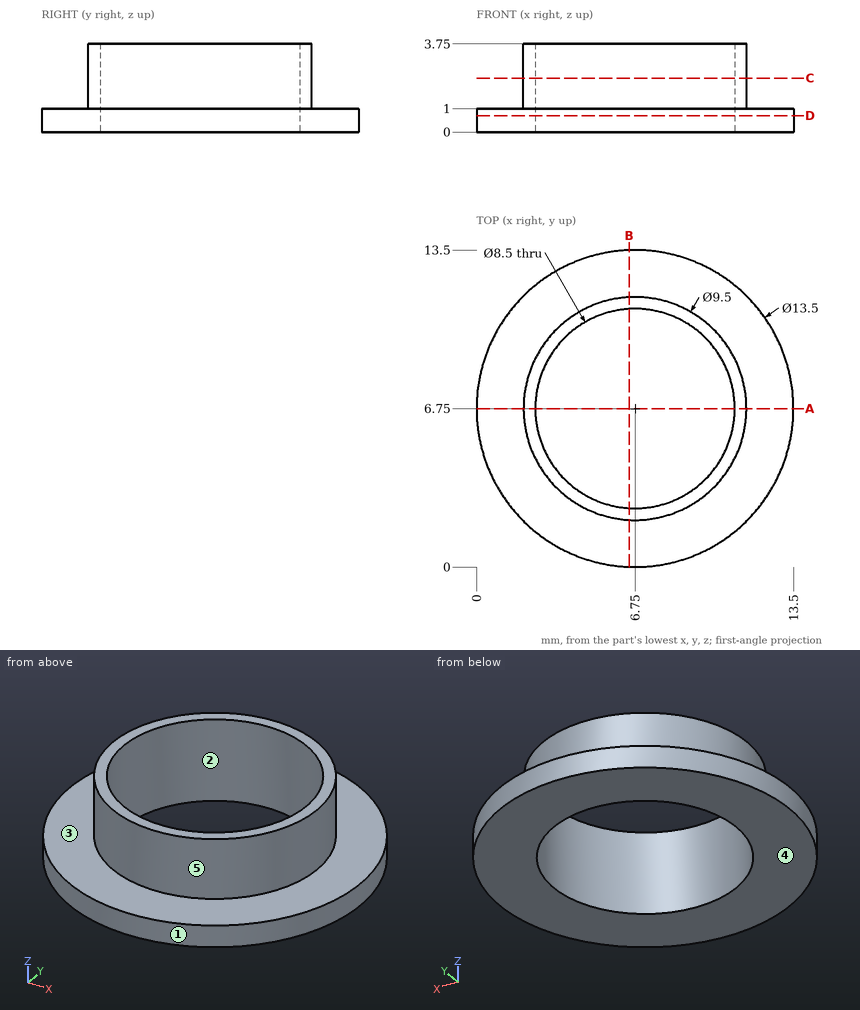
Source: three-view drawing plus pictorial views. Frame: mm from the lowest corner of the part. A direction names the side the tool comes from. Give positions to 0.01 mm unless a question says otherwise; leave off trailing zeros. Write each loop counter-clockwise with the first axis right and the second up, starting at its lowest first coordinate (ties: lowest second). Pieces come first, ordered by that corner, then holes. Notation, with made-up numbers: (78.25, -16) - (112.25, -16) arc R19 ccw to (112.25, 6) - close; hole circle Ø10 at (66.25, -36). An arc over 180 degrees is marked (long way). Write item = value, one per line. Start each with the question number.
Q1. Material intervals for probe 1 along X at (y, z) = (6.75, 1.3); probe 2 along Y at (x, z) = (6.75, 0.95), sorted ascending.
Q2. Cut plane C-C, the plane z = 2.3. Return loops of the section in (x, y).
Q3. Cut plane B-B, the plane x = 6.5. Return loops of the section in (y, z), then the cut area to 3 significant figures.
Q4. Cut plane D-D, the plane z = 0.7. Return loops of the section in (x, y), then the cut area to 3 significant figures.
Q5. Cut plane A-A, the plane y = 6.75. Return loops of the section in (x, z).
Q6. Draft query along Y for the marked faces 1, 2 and 3. Return one class per face: +Y half, -Y half, draft (parallel to the pull), parting line (faces both ways), or undercut.
Q7. Reachability of the marked faces 4 and 5 from +Z, -Z, +X, -X, +Y, -Y: full face, straight path, thin tool, end or side. Return the list, or none.
Computed values:
q1.probe_1 = 2 to 2.5, 11 to 11.5
q1.probe_2 = 0 to 2.5, 11 to 13.5
q2.outline = circle Ø9.5 at (6.75, 6.75); hole circle Ø8.5 at (6.75, 6.75)
q3.outline = (0, 0) - (2.51, 0) - (2.51, 3.75) - (2.01, 3.75) - (2.01, 1) - (0, 1) - close; (10.99, 0) - (13.5, 0) - (13.5, 1) - (11.49, 1) - (11.49, 3.75) - (10.99, 3.75) - close
q3.area = 7.76 mm²
q4.outline = circle Ø13.5 at (6.75, 6.75); hole circle Ø8.5 at (6.75, 6.75)
q4.area = 86.4 mm²
q5.outline = (0, 0) - (2.5, 0) - (2.5, 3.75) - (2, 3.75) - (2, 1) - (0, 1) - close; (11, 0) - (13.5, 0) - (13.5, 1) - (11.5, 1) - (11.5, 3.75) - (11, 3.75) - close
q6.face_1 = parting line
q6.face_2 = undercut
q6.face_3 = draft
q7.face_4 = -Z, +X, -X, +Y, -Y
q7.face_5 = +Z
